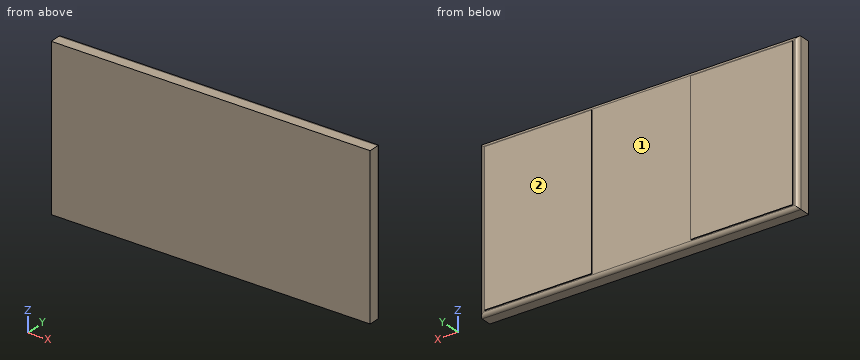
```python
from build123d import *

# Parameters (mm, degrees)
SKETCH1_W           = 2286
SKETCH1_H           = 1143
BOSS_EXTRUDE1_DEPTH = 101.6
SKETCH2_W           = 730.915860416
SKETCH2_H           = 1078.506958481
SKETCH2_W_2         = 767.684139584
CUT_EXTRUDE1_DEPTH  = 88.9
SKETCH3_W           = 730.915860416
SKETCH3_H           = 1078.506958481
SKETCH3_W_2         = 767.684139584
BOSS_EXTRUDE2_DEPTH = 93.98
FILLET1_R           = 25.4


with BuildPart() as part:
    # Sketch1 → Boss-Extrude1 (new body)
    with BuildSketch(Plane(origin=(0, 0, 0), x_dir=(1, 0, 0), z_dir=(0, 1, 0))):
        with Locations((1143, 571.5)):
            Rectangle(SKETCH1_W, SKETCH1_H)
    extrude(amount=BOSS_EXTRUDE1_DEPTH)

    # Sketch2 → Cut-Extrude1 (cut)
    with BuildSketch(Plane(origin=(0, 101.6, 0), x_dir=(1, 0, 0), z_dir=(0, 1, 0))):
        with Locations((403.557930208, 571.468483779)):
            Rectangle(SKETCH2_W, SKETCH2_H)
        with Locations((1864.057930208, 571.468483779)):
            Rectangle(SKETCH2_W_2, SKETCH2_H)
    extrude(amount=-CUT_EXTRUDE1_DEPTH, mode=Mode.SUBTRACT)

    # Sketch3 → Boss-Extrude2 (add)
    with BuildSketch(Plane(origin=(0, 12.7, 0), x_dir=(1, 0, 0), z_dir=(0, 1, 0))):
        with Locations((403.557930208, 571.468483779)):
            Rectangle(SKETCH3_W, SKETCH3_H)
        with Locations((1864.057930208, 571.468483779)):
            Rectangle(SKETCH3_W_2, SKETCH3_H)
    extrude(amount=BOSS_EXTRUDE2_DEPTH)

    # Fillet1
    fillet1_edges = [part.edges().sort_by_distance(p)[0] for p in [
        (2286, 101.6, -571.5),
        (1143, 101.6, -1143),
        (0, 101.6, -571.5),
        (1143, 101.6, 0),
    ]]
    fillet(fillet1_edges, radius=FILLET1_R)


solid = part.part
```
Design review of the part built by this model. Coordinates are the model's own, in mm. Face numbers are marked on the shaded views. Coordinates: 2 decimals unless noted, no trailing zeros. Order: outer loops, then holes, each group sorted by start corner. A loop starts at its lowest first (then second) coordinate and runs counter-clockwise, first axis right, second up.
1) Take a section at B-B, the plane x = 929.5. Give the boundary of the cut face in (y, z).
2) Wall thickness on line 1 along Y through (x, z) = (874, -716.5); line 2 along Z through (x, y) = (1395, 77.5); line 3 along X through (y, z) = (88, -848): over which ranges is each line inside the solid? List them lowest first.
3) Clearance check with flat-ended pins moving along their axes: pin 1 (4 mm diameter, centred on x = 279, y = 104.5, fed in from -Z); pin 2 (8 mm diameter, centred on x = 859.5, y = 83.5, fed in from +Z); pin 3 (2.5 mm diameter, centred on y = 103, z = -513.5, fed in from -X). State where each tip first meets the part, or that it passes through.
4) Take a section at A-A, the plane z = -513. Give the boundary of the cut face in (x, y).
5) Mouldability with a two-part tool opening along X and no side actions: class the marked faces 1 and 2 as +X half, -X half, draft (parallel to the pull), parting line (faces both ways), or undercut.
Returned:
1. outline: (0, -1143) - (76.2, -1143) arc R25.4 ccw to (101.6, -1117.6) - (101.6, -25.4) arc R25.4 ccw to (76.2, 0) - (0, 0) - close
2. line 1: y = 0 to 101.6
2. line 2: z = -1142.97 to -0.03
2. line 3: x = 2.91 to 2283.09
3. pin 1: stops at z = -1110.72
3. pin 2: stops at z = -0.22
3. pin 3: stops at x = 38.1
4. outline: (0, 0) - (2286, 0) - (2286, 76.2) arc R25.4 ccw to (2260.6, 101.6) - (2247.9, 101.6) - (2247.9, 106.68) - (1480.22, 106.68) - (1480.22, 101.6) - (769.02, 101.6) - (769.02, 106.68) - (38.1, 106.68) - (38.1, 101.6) - (25.4, 101.6) arc R25.4 ccw to (0, 76.2) - close
5. face 1: undercut
5. face 2: draft
